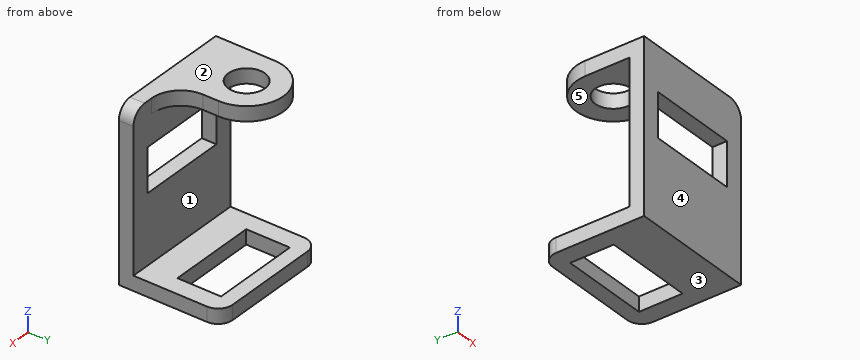
```python
from build123d import *

# Parameters (mm, degrees)
SKETCH1_W            = 55
SKETCH1_H            = 74.202
SKETCH1_W_2          = 39
SKETCH1_H_2          = 19
BOSS_EXTRUDE1_DEPTH  = 6.35
SKETCH2_W            = 55
SKETCH2_H            = 38.35
SKETCH2_W_2          = 39
SKETCH2_H_2          = 19
BOSS_EXTRUDE2_DEPTH  = 6.35
SKETCH12_R           = 7.9375
BOSS_EXTRUDE11_DEPTH = 6.35
FILLET2_R            = 12.7
FILLET1_R            = 6.35


with BuildPart() as part:
    # Sketch1 → Boss-Extrude1 (new body)
    with BuildSketch(Plane(origin=(0, 0, 0), x_dir=(1, 0, 0), z_dir=(0, 1, 0))):
        with Locations((0, 8.601)):
            Rectangle(SKETCH1_W, SKETCH1_H)
        Rectangle(SKETCH1_W_2, SKETCH1_H_2, mode=Mode.SUBTRACT)
    extrude(amount=BOSS_EXTRUDE1_DEPTH)

    # Sketch2 → Boss-Extrude2 (add)
    with BuildSketch(Plane.XY.offset(-45.702)):
        with Locations((0, 25.525)):
            Rectangle(SKETCH2_W, SKETCH2_H)
        with Locations((0, 28.85)):
            Rectangle(SKETCH2_W_2, SKETCH2_H_2, mode=Mode.SUBTRACT)
    extrude(amount=BOSS_EXTRUDE2_DEPTH)

    # Sketch12 → Boss-Extrude11 (add)
    with BuildSketch(Plane.XY.offset(28.5)):
        with BuildLine():
            Line((-27.5, 25.68), (-27.5, 6.35))
            Line((-27.5, 6.35), (4.5, 6.35))
            Line((4.5, 6.35), (4.5, 25.68))
            ThreePointArc((4.5, 25.68), (-11.5, 41.68), (-27.5, 25.68))
        make_face()
        with Locations((-11.5, 25.68)):
            Circle(SKETCH12_R, mode=Mode.SUBTRACT)
    extrude(amount=-BOSS_EXTRUDE11_DEPTH)

    # Fillet2
    fillet2_edges = [part.edges().sort_by_distance(p)[0] for p in [
        (4.5, 6.35, 25.325),
    ]]
    fillet(fillet2_edges, radius=FILLET2_R)

    # Fillet1
    fillet1_edges = [part.edges().sort_by_distance(p)[0] for p in [
        (27.5, 44.7, -42.527),
        (-27.5, 44.7, -42.527),
        (27.5, 3.175, 28.5),
    ]]
    fillet(fillet1_edges, radius=FILLET1_R)


solid = part.part
```
Work out the finished part from the listing and answer in its coordinate system (mm). Face numbers are marked on the shaded views. A direction names the side the tool comes from. Round coordinates to 2 decimals unless told otherwise and drop trailing zeros. Write each loop counter-clockwise with the first axis right and the second up, starting at its lowest first coordinate (ties: lowest second). Pieces come first, ordered by that corner, then holes. Notation, with made-up numbers: (36, 66) - (91, 66) arc R28 cw to (91, 100) - close; hole circle Ø4 at (75, -12). An arc over 180 degrees is marked (long way). Return JSON: item names as keys, results as strings. Group by question number.
Q1. For the marked faces 4 and 5, determine the directions among +Z, -Z, +X, -X, +Y, -Y from which every point of the face is accessible in a straight line to the end or side of a thin tool.
Q2. The part is cut by section D-D on y = 31. Write down the section's boundary in (x, z).
Q3. The part is cut by section A-A on x = -11.5. Write down the section's boundary in (y, z).
Q4. Find the intervals of material crossed by L1, parallel to Y at x = -11.5, z = 24; L2, parallel to Z at x = -17, y = 14; L3, parallel to Y at x = -11, z = 25, in increasing order.
Q5. The mould has two halves that part along Z. Classify the marked faces 1, 2 and 3: released by +Z, released by -Z, zero draft, split by the parting line, or undercut.
Q6. The part is cut by section C-C on y = 9. Write down the section's boundary in (x, z), then the cut area to 3 significant figures.
Q7. Each of these flat-tipped pins is pushed along its axis until it touches: pin 1 Ø5 at (x, z) = (18, -17.5) entering from +Y; pin 2 Ø9.5 at (x, y) = (-11.5, 25.68) entering from +Z; pin 3 Ø1.9 at (y, z) = (24, 24.5) entering from +X. Where does it stop, or does it pass through?
Q8. The part is cut by section B-B on z = -8. Write down the section's boundary in (x, y).
Solved:
{
 "1": {"face 4": "+Z, -Z, +X, -X, -Y", "face 5": "+X, -X, +Y"},
 "2": {"outline": "(-27.5, -45.7) - (-19.5, -45.7) - (-19.5, -39.35) - (-27.5, -39.35) - close; (-26.59, 22.15) - (-17.39, 22.15) - (-17.39, 28.5) - (-26.59, 28.5) - close; (-5.61, 22.15) - (3.59, 22.15) - (3.59, 28.5) - (-5.61, 28.5) - close; (19.5, -45.7) - (27.5, -45.7) - (27.5, -39.35) - (19.5, -39.35) - close"},
 "3": {"outline": "(0, -45.7) - (19.35, -45.7) - (19.35, -39.35) - (6.35, -39.35) - (6.35, -9.5) - (0, -9.5) - close; (0, 9.5) - (6.35, 9.5) - (6.35, 22.15) - (17.74, 22.15) - (17.74, 28.5) - (0, 28.5) - close; (33.62, 22.15) - (41.68, 22.15) - (41.68, 28.5) - (33.62, 28.5) - close; (38.35, -45.7) - (44.7, -45.7) - (44.7, -39.35) - (38.35, -39.35) - close"},
 "4": {"L1": "0 to 17.74, 33.62 to 41.68", "L2": "-45.7 to -39.35, 22.15 to 28.5", "L3": "0 to 17.76, 33.6 to 41.67"},
 "5": {"face 1": "undercut", "face 2": "released by +Z", "face 3": "released by -Z"},
 "6": {"outline": "(-27.5, -45.7) - (27.5, -45.7) - (27.5, -39.35) - (-27.5, -39.35) - close; (-27.5, 22.15) - (9.44, 22.15) - (9.44, 28.5) - (-27.5, 28.5) - close", "area": "584 mm²"},
 "7": {"pin 1": "y = 6.35", "pin 2": "through", "pin 3": "x = 4.5"},
 "8": {"outline": "(-27.5, 0) - (-19.5, 0) - (-19.5, 6.35) - (-27.5, 6.35) - close; (19.5, 0) - (27.5, 0) - (27.5, 6.35) - (19.5, 6.35) - close"}
}
